```python
from build123d import *

# Parameters (mm, degrees)
BOSS_EXTRUDE1_DEPTH = 1
SKETCH2_W           = 3.3
SKETCH2_H           = 15
BOSS_EXTRUDE2_DEPTH = 1
SKETCH3_W           = 1.6
SKETCH3_H           = 5
BOSS_EXTRUDE3_DEPTH = 1.2
SKETCH4_W           = 1.6
SKETCH4_H           = 1.2
BOSS_EXTRUDE4_DEPTH = 1.2


with BuildPart() as part:
    # Sketch1 → Boss-Extrude1 (new body)
    with BuildSketch(Plane(origin=(0, 0, 0), x_dir=(1, 0, 0), z_dir=(0, 1, 0))):
        with BuildLine():
            Line((-4.5, -0.75), (-4.5, -9.8))
            Line((-4.5, -9.8), (4.5, -9.8))
            Line((4.5, -9.8), (4.5, -0.75))
            Line((4.5, -0.75), (3.65, -0.75))
            ThreePointArc((3.65, -0.75), (2.9, 0), (3.65, 0.75))
            Line((3.65, 0.75), (4.5, 0.75))
            Line((4.5, 0.75), (4.5, 9.8))
            Line((4.5, 9.8), (-4.5, 9.8))
            Line((-4.5, 9.8), (-4.5, 0.75))
            Line((-4.5, 0.75), (-3.65, 0.75))
            ThreePointArc((-3.65, 0.75), (-3.119669914, 0.530330086), (-2.9, 0))
            ThreePointArc((-2.9, 0), (-3.119669914, -0.530330086), (-3.65, -0.75))
            Line((-3.65, -0.75), (-4.5, -0.75))
        make_face()
    extrude(amount=BOSS_EXTRUDE1_DEPTH)

    # Sketch2 → Boss-Extrude2 (add)
    with BuildSketch(Plane(origin=(0, 1, 0), x_dir=(1, 0, 0), z_dir=(0, 1, 0))):
        Rectangle(SKETCH2_W, SKETCH2_H)
    extrude(amount=BOSS_EXTRUDE2_DEPTH)

    # Sketch3 → Boss-Extrude3 (add)
    with BuildSketch(Plane(origin=(0, 1, 0), x_dir=(1, 0, 0), z_dir=(0, 1, 0))):
        with Locations((-3.7, -7.3)):
            Rectangle(SKETCH3_W, SKETCH3_H)
        with Locations((3.7, -7.3)):
            Rectangle(SKETCH3_W, SKETCH3_H)
    extrude(amount=BOSS_EXTRUDE3_DEPTH)

    # Sketch4 → Boss-Extrude4 (add)
    with BuildSketch(Plane.XY.offset(9.8)):
        with Locations((-3.7, 1.6)):
            Rectangle(SKETCH4_W, SKETCH4_H)
        with Locations((3.7, 1.6)):
            Rectangle(SKETCH4_W, SKETCH4_H)
    extrude(amount=BOSS_EXTRUDE4_DEPTH)


solid = part.part
```
CAD build for the part. Positions are in the model's coordinates, mm. A direction names the side the tool comes from. Coordinates: 2 decimals unless noted, no trailing zeros. Order: outer loops, then holes, each group sorted by start corner. A loop starts at its lowest first (then second) coordinate and runs counter-clockwise, first axis right, second up. Notation, with made-up numbers: M 9.25,76 L 43.25,76 A12 ccw 43.25,87 Z; hole C 49,-38.75 d2. An arc over 180 degrees is marked long. Answer as CSV lines item,"result".
1) Cut at A-A (x = -4). List the corners of the cut face in (y, z).
Verdict:
outline,"M 0,-9.8 L 1,-9.8 L 1,-0.75 L 0,-0.75 Z; M 0,0.75 L 1,0.75 L 1,4.8 L 2.2,4.8 L 2.2,11 L 1,11 L 1,9.8 L 0,9.8 Z"
2) Cut at D-D (x = 1). List the corners of the cut face in (y, z).
Verdict:
outline,"M 0,-9.8 L 1,-9.8 L 1,-7.5 L 2,-7.5 L 2,7.5 L 1,7.5 L 1,9.8 L 0,9.8 Z"
3) Flat gauge pins, fed straight in: P1, Ø1, axis at x = 4, z = 10.5, coming from the -Y side; P2, Ø1.3, axis at x = 3.5, y = 1.5, coming from the -Z side; P3, Ø1, axis at x = -2, z = -6, coming from the +Y side; P4, Ø1, axis at x = -1.5, y = 1, coming from the +Z side. Where does each tip first touch, or does it go through?
Verdict:
P1,"y = 1"
P2,"z = -9.8"
P3,"y = 2"
P4,"z = 9.8"
4) Cut at C-C (z = 9.5). List the corners of the cut face in (x, y), then the cut area to 3 significant figures.
Verdict:
outline,"M -4.5,0 L 4.5,0 L 4.5,2.2 L 2.9,2.2 L 2.9,1 L -2.9,1 L -2.9,2.2 L -4.5,2.2 Z"
area,"12.8 mm2"
5) 3-axis set-ups, long thin cutter, end or side, ignore diameter. For faces 1 (the flat face through (-4.5, 0.5, -5.3)), 2 (the flat face through (-4, 1, 10)), 3 (the flat face through (1.65, 1.5, 0.1)), 4 (the flat face through (4, 2, 4.8)), 5 (the flat face through (4.5, 1, 6)): which of +Z, -Z, +X, -X, +Y, -Y reach the whole face in a straight line?
Verdict:
face 1,"+Z, -Z, -X, +Y, -Y"
face 2,"+Z, +X, -X, -Y"
face 3,"+Z, -Z, +Y"
face 4,"-Z, +X, +Y"
face 5,"+Z, -Z, +X, +Y, -Y"
6) Drill centre lines: L1, parallel to Y at x = -2.5, z = 9; L2, parallel to X at y = 1.9, z = -7.25; L3, parallel to Z at x = 2, y = 0.35. Where is each one in solid material? Low to high. Write a range as from..to.
Verdict:
L1,"0..1"
L2,"-1.65..1.65"
L3,"-9.8..9.8"
7) Cut at B-B (y = 0.4). List the corners of the cut face in (x, z).
Verdict:
outline,"M -4.5,-9.8 L 4.5,-9.8 L 4.5,-0.75 L 3.65,-0.75 A0.75 cw 3.65,0.75 L 4.5,0.75 L 4.5,9.8 L -4.5,9.8 L -4.5,0.75 L -3.65,0.75 A0.75 cw -3.65,-0.75 L -4.5,-0.75 Z"
8) Mould opens along Z. For faces 6 (the flat face through (-4.1, 0.5, 0.75)), 7 (the flat face through (-1.65, 1.5, 0.1)), 8 (the flat face through (-4, 2, 4.8)) say: released by +Z, released by -Z, zero draft, split by the parting line, or undercut.
Verdict:
face 6,"undercut"
face 7,"zero draft"
face 8,"released by -Z"
